Input: part model. Units: mm. Frame: model coordinates. Face numbers are marked on the shaded views. A direction names the side the tool comes from. Coordinates: 2 decimals unless noted, no trailing zeros. Write each loop counter-clockwise with the first axis right and the second up, starting at its lowest first coordinate (ties: lowest second). Pieces come first, ordered by that corner, then holes. Notation, with made-up numbers: M 30.5,76.5 L 81.5,76.5 A30 ccw 81.5,111.5 Z; hole C 78,-4 d7. An arc over 180 degrees is marked long. Answer as a JSON object with one key per item and string values. Group by question number.
from build123d import *

# Parameters (mm, degrees)
SKETCH1_W           = 38.1
SKETCH1_H           = 38.1
BOSS_EXTRUDE1_DEPTH = 64.389
SKETCH2_W           = 8.720666582
SKETCH2_H           = 12.954
CUT_EXTRUDE1_DEPTH  = 38.1
SKETCH3_W           = 38.1
SKETCH3_H           = 38.1
BOSS_EXTRUDE2_DEPTH = 25.4
SKETCH1_3_W         = 25.908
SKETCH1_3_H         = 25.908
CUT_EXTRUDE2_DEPTH  = 70.739
CUT_EXTRUDE4_DEPTH  = 32.004
SKETCH7_W           = 38.1
SKETCH7_H           = 25.4
BOSS_EXTRUDE3_DEPTH = 20.066
SKETCH9_W           = 11.43
SKETCH9_H           = 13.716
CUT_EXTRUDE5_DEPTH  = 21.59
FILLET1_R           = 2.54


with BuildPart() as part:
    # Sketch1 → Boss-Extrude1 (new body)
    with BuildSketch(Plane(origin=(0, 0, 0), x_dir=(1, 0, 0), z_dir=(0, 1, 0))):
        Rectangle(SKETCH1_W, SKETCH1_H)
    extrude(amount=BOSS_EXTRUDE1_DEPTH)

    # Sketch2 → Cut-Extrude1 (cut)
    with BuildSketch(Plane.XY.offset(19.05)):
        with Locations((8.339666836, 16.637)):
            Rectangle(SKETCH2_W, SKETCH2_H)
        with Locations((-8.339666709, 16.637)):
            Rectangle(SKETCH2_W, SKETCH2_H)
    extrude(amount=-CUT_EXTRUDE1_DEPTH, mode=Mode.SUBTRACT)

    # Sketch3 → Boss-Extrude2 (add)
    with BuildSketch(Plane(origin=(0, 64.389, 0), x_dir=(-1, 0, 0), z_dir=(0, -1, 0))):
        Rectangle(SKETCH3_W, SKETCH3_H)
    extrude(amount=-BOSS_EXTRUDE2_DEPTH)

    # Sketch1<3> → Cut-Extrude2 (cut)
    with BuildSketch(Plane(origin=(0, 0, 0), x_dir=(1, 0, 0), z_dir=(0, 1, 0))):
        Rectangle(SKETCH1_3_W, SKETCH1_3_H)
    extrude(amount=CUT_EXTRUDE2_DEPTH, mode=Mode.SUBTRACT)

    # Sketch5 → Cut-Extrude4 (cut)
    with BuildSketch(Plane(origin=(19.05, 0, 0), x_dir=(0, 0, -1), z_dir=(1, 0, 0))):
        Polygon((-12.7, 80.264), (12.7, 80.264), (12.7, 73.914), (6.35, 73.914), (6.35, 64.389), (-6.35, 64.389), (-6.35, 73.914), (-12.7, 73.914), align=None)
    extrude(amount=-CUT_EXTRUDE4_DEPTH, mode=Mode.SUBTRACT)

    # Sketch7 → Boss-Extrude3 (add)
    with BuildSketch(Plane.XY.offset(19.05)):
        with Locations((0, 77.089)):
            Rectangle(SKETCH7_W, SKETCH7_H)
    extrude(amount=BOSS_EXTRUDE3_DEPTH)

    # Sketch9 → Cut-Extrude5 (cut)
    with BuildSketch(Plane(origin=(0, 89.789, 0), x_dir=(1, 0, 0), z_dir=(0, 1, 0))):
        with Locations((6.985, -25.908)):
            Rectangle(SKETCH9_W, SKETCH9_H)
    extrude(amount=-CUT_EXTRUDE5_DEPTH, mode=Mode.SUBTRACT)

    # Fillet1
    fillet1_edges = [part.edges().sort_by_distance(p)[0] for p in [
        (19.05, 32.1945, 19.05),
        (-19.05, 32.1945, 19.05),
        (0, 64.389, 19.05),
        (-19.05, 64.389, 29.083),
        (19.05, 64.389, 29.083),
        (-19.05, 77.089, 39.116),
        (0, 64.389, 39.116),
        (19.05, 77.089, 39.116),
        (0, 0, 19.05),
        (19.05, 0, 0),
        (0, 0, -19.05),
        (-19.05, 0, 0),
        (19.05, 44.8945, -19.05),
        (-19.05, 44.8945, -19.05),
    ]]
    fillet(fillet1_edges, radius=FILLET1_R)


solid = part.part
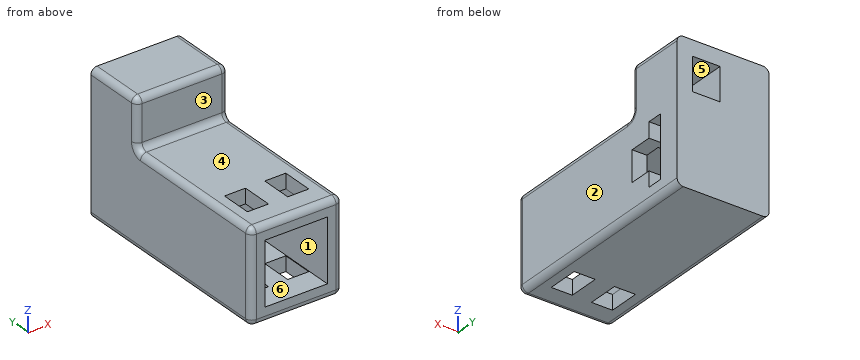
Q1. Section B-B, the plane x = 14. Return the cut outline in (y, z), and give its area (3 significant figures).
Q2. Draft query along X for the marked faces 1, 2 and 3. Return one class per face: released by +X, released by -X, zero draft, split by the parting line, or undercut.
Q3. Line query: line 1 (X direction, y = 20, z = 13.5); line 2 (Z direction, x = 7, y = 75); line 3 (X direction, y = 36, z = 5). Output: solid intervals per line, ascending. Write a range as from..to.
Q4. Section D-D, the plane x = -15. Return the cut outline in (y, z).
Q5. Pin query (flat end, axial travel): pin 1 Ø2 at (x, z) = (9.5, -9) entering from -Y; pin 2 Ø4 at (x, z) = (-1.5, 30) entering from -Y. Return the tip coordinate at first contact, or that it passes through.
Q6. Section A-A, the plane x = 9. State how many separate pieces and enclosed holes the cut face has, and give its area (3 significant figures).
Q7. Access query for the marked faces 4, 5 and 6. Directions: +Z, -Z, +X, -X, +Y, -Y. A direction counts if a zero-diameter tool reaches every point of the face in a straight line with its end or side. Return the directions, or none.
Q8. Section C-C, the plane z = -15. Return the cut outline in (x, y), and give its area (3 significant figures).
Filled in:
{
 "1": {"outline": "M 0,-16.51 A2.54 ccw 2.54,-19.05 L 89.79,-19.05 L 89.79,39.12 L 66.93,39.12 A2.54 ccw 64.39,36.58 L 64.39,21.59 A2.54 cw 61.85,19.05 L 2.54,19.05 A2.54 ccw 0,16.51 Z; hole M 64.39,-6.35 L 73.91,-6.35 L 73.91,-12.7 L 80.26,-12.7 L 80.26,12.7 L 73.91,12.7 L 73.91,6.35 L 64.39,6.35 Z", "area": "3,650 mm^2"},
 "2": {"face 1": "undercut", "face 2": "released by +X", "face 3": "zero draft"},
 "3": {"line 1": "-19.05..-12.7, -3.98..3.98, 12.7..19.05", "line 2": "-19.05..-12.7, 12.7..19.05, 32.77..39.12", "line 3": "-19.05..-12.95, 12.95..19.05"},
 "4": {"outline": "M 0,-16.51 A2.54 ccw 2.54,-19.05 L 89.79,-19.05 L 89.79,39.12 L 66.93,39.12 A2.54 ccw 64.39,36.58 L 64.39,21.59 A2.54 cw 61.85,19.05 L 2.54,19.05 A2.54 ccw 0,16.51 Z"},
 "5": {"pin 1": "y = 70.74", "pin 2": "y = 64.39"},
 "6": {"separate pieces": "3", "enclosed holes": "0", "area": "1,440 mm^2"},
 "7": {"face 4": "+Z, +X, -X, -Y", "face 5": "+Y", "face 6": "-Y"},
 "8": {"outline": "M -19.05,2.54 A2.54 ccw -16.51,0 L 16.51,0 A2.54 ccw 19.05,2.54 L 19.05,89.79 L -19.05,89.79 Z; hole M -12.7,10.16 L -3.98,10.16 L -3.98,23.11 L -12.7,23.11 Z; hole M 3.98,10.16 L 12.7,10.16 L 12.7,23.11 L 3.98,23.11 Z", "area": "3,190 mm^2"}
}
